The listing builds one solid part. Answer for the finished solid, in the listing's coordinates (mm). A direction names the side the tool comes from. Give positions to 0.01 mm unless a question says otherwise; leave off trailing zeros. Order: outer loops, then holes, each group sorted by start corner. A loop starts at its lowest first (then second) coordinate and runs counter-clockwise, first axis right, second up. Notation, with made-up numbers: (29, 19.5) - (51, 19.5) arc R18 cw to (51, 42.5) - close; hole circle Ø11 at (76.25, -19.5). An arc over 180 degrees is marked (long way). Answer as a JSON object with one key per item and string values. Group by question number.
Q1. A cutting plane is placed at B-B, the plane x = 35.5. Give the vertices of the cut face in (y, z), and give its area (3 significant figures).
Q2. A cutting plane is placed at D-D, the plane x = 7.5. Give the vertices of the cut face in (y, z), and give its area (3 significant figures).
Q3. The mould has two halves that part along Y. Classify faces 1 (the face through (6.4, 95.3, 200.4)), 2 (the face through (0, 50, 200)), 3 (the face through (12.7, 50, 200)), 4 (the face through (95.3, 6.4, 200.4)): released by +Y, released by -Y, zero draft, split by the parting line, or undercut.
Q4. For faces 5 (the face through (82.6, 19.1, 200.4)), 6 (the face through (101.6, 50, 200)), determine the directions among +Z, -Z, +X, -X, +Y, -Y from which every point of the face is accessible in a straight line to the end or side of a thin tool.
Q5. A cutting plane is placed at C-C, the plane z = 187.5. Give the vertices of the cut face in (x, y), and give its area (3 significant figures).
Q6. A cutting plane is placed at A-A, the plane y = 21. Give the vertices of the cut face in (x, z).
Q7. Consider line 1 (Y direction, x = 37, z = 88); line 2 (Y direction, x = 81.5, z = 27). Determine where each line is inside the solid, lowest interval first.
from build123d import *

# Parameters (mm, degrees)
F0_W     = 101.6
F0_H     = 101.6
F0_W_2   = 76.2
F0_H_2   = 76.2
F1_DEPTH = 406.4
F2_SIZE  = 12.7
F3_SIZE  = 12.7


with BuildPart() as f1:
    # F0 (on Top) → F1 (new body)
    with BuildSketch(Plane.XY):
        with Locations((50.8, 50.8)):
            Rectangle(F0_W, F0_H)
        with Locations((50.8, 50.8)):
            Rectangle(F0_W_2, F0_H_2, mode=Mode.SUBTRACT)
    extrude(amount=F1_DEPTH)

    # F2
    f2_edges = [f1.edges().sort_by_distance(p)[0] for p in [
        (12.7, 88.9, 203.2),
        (88.9, 88.9, 203.2),
        (88.9, 12.7, 203.2),
        (12.7, 12.7, 203.2),
    ]]
    chamfer(f2_edges, length=F2_SIZE)

    # F3
    f3_edges = [f1.edges().sort_by_distance(p)[0] for p in [
        (101.6, 0, 203.2),
        (101.6, 101.6, 203.2),
        (0, 0, 203.2),
        (0, 101.6, 203.2),
    ]]
    chamfer(f3_edges, length=F3_SIZE)


solid = f1.part
Reply:
{
 "1": {"outline": "(0, 0) - (12.7, 0) - (12.7, 406.4) - (0, 406.4) - close; (88.9, 0) - (101.6, 0) - (101.6, 406.4) - (88.9, 406.4) - close", "area": "10,300 mm^2"},
 "2": {"outline": "(5.2, 0) - (96.4, 0) - (96.4, 406.4) - (5.2, 406.4) - close", "area": "37,100 mm^2"},
 "3": {"face 1": "released by +Y", "face 2": "zero draft", "face 3": "undercut", "face 4": "released by -Y"},
 "4": {"face 5": "+Z, -Z", "face 6": "+Z, -Z, +X, +Y, -Y"},
 "5": {"outline": "(0, 12.7) - (12.7, 0) - (88.9, 0) - (101.6, 12.7) - (101.6, 88.9) - (88.9, 101.6) - (12.7, 101.6) - (0, 88.9) - close; hole (12.7, 25.4) - (25.4, 12.7) - (76.2, 12.7) - (88.9, 25.4) - (88.9, 76.2) - (76.2, 88.9) - (25.4, 88.9) - (12.7, 76.2) - close", "area": "4,520 mm^2"},
 "6": {"outline": "(0, 0) - (17.1, 0) - (17.1, 406.4) - (0, 406.4) - close; (84.5, 0) - (101.6, 0) - (101.6, 406.4) - (84.5, 406.4) - close"},
 "7": {"line 1": "y = 0 to 12.7, 88.9 to 101.6", "line 2": "y = 0 to 18, 83.6 to 101.6"}
}
